Can you work these out from the model? Positions are in its coordinate system, mm. A direction names the side the tool comes from. Coordinates: 2 decimals unless noted, no trailing zeros. Answer as a JSON object with one key per item and string values. Group by question number.
Item 1: Which directions (+Z, -Z, +X, -X, +Y, -Y) give clear straight access to the entire face, cutting with the end or side of a thin tool? Please do faces 4 (the flat face through (0, -62, 0.25)), 5 (the flat face through (-4.5, -2, 0)).
Item 2: We'd pull the mould along Y, two halves only. Please class faces 1 (the flat face through (2, -120, 0.25)), 2 (the flat face through (0, 150, 0)), 3 (the flat face through (0, -2, -3.25)): +Y half, -Y half, draft (parallel to the pull), parting line (faces both ways), or undercut.
Item 3: I'm going to push flat-ended pins straight in: pin 1 Ø5 at (x, y) = (0, -60) entering from -Z; pin 2 Ø2 at (x, y) = (0, 80) entering from -Z. Where does each tip first touch, or does it pass through?
Item 4: If I drill on line 1 (X direction, y = -140, z = -0.8); line 2 (X direction, y = -59, z = -1.5), over which ranges is the centre line in solid material (lowest first)?
Item 5: Suppose I cut it at A-A (z = 1.75). Count the separate pieces of the cut face and the enclosed holes in it, then the cut area to 3 significant figures.
```python
from build123d import *

# Parameters (mm, degrees)
F0_W           = 9
F0_H           = 6.5
F1_DEPTH       = 150
F1_DEPTH_BACK  = 150
F3_D           = 3.5
F3_CBORE_D     = 6
F3_CBORE_DEPTH = 3


with BuildPart() as f1:
    # F0 (on Front) → F1 (new body, two sides)
    with BuildSketch(Plane.XZ) as f1_sk:
        Rectangle(F0_W, F0_H)
    extrude(amount=F1_DEPTH)
    extrude(f1_sk.sketch, amount=-F1_DEPTH_BACK)

    # F3 (through all)
    with Locations(Plane.XY.offset(3.25)):
        with Locations((0, -140), (0, -120), (0, -100), (0, -80), (0, -60), (0, -40), (0, -20), (0, 0), (0, 20), (0, 40), (0, 60), (0, 80), (0, 100), (0, 120), (0, 140)):
            CounterBoreHole(F3_D / 2, F3_CBORE_D / 2, F3_CBORE_DEPTH)


solid = f1.part
```
From the geometry:
{
 "1": {"face 4": "+Z", "face 5": "+Z, -Z, -X, +Y, -Y"},
 "2": {"face 1": "undercut", "face 2": "+Y half", "face 3": "draft"},
 "3": {"pin 1": "z = -3.25", "pin 2": "through"},
 "4": {"line 1": "-4.5 to -1.75, 1.75 to 4.5", "line 2": "-4.5 to -1.44, 1.44 to 4.5"},
 "5": {"separate pieces": "1", "enclosed holes": "15", "area": "2,280 mm2"}
}
